Autodesk Inventor part; units mm, degrees
ref_plane "YZ Plane" through (0, 0, 0) normal (1, 0, 0) x (0, 1, 0)
ref_plane "XZ Plane" through (0, 0, 0) normal (0, 1, 0) x (-1, 0, 0)
ref_plane "XY Plane" through (0, 0, 0) normal (0, 0, 1) x (1, 0, 0)
sketch "Sketch1" plane through (0, 0, 0) normal (0, 0, 1) x (1, 0, 0)
  circle A0 centre (0, 0) radius 11.5
  circle A1 centre (-15.5, 15.5) radius 1.5
  circle A2 centre (-15.5, -15.5) radius 1.5
  circle A3 centre (15.5, 15.5) radius 1.5
  circle A4 centre (15.5, -15.5) radius 1.5
  line L0 (-21, -24) -> (21, -24)
  line L1 (0, 20) -> (4.5462, 20) construction
  line L2 (-21, 21) -> (-1, 21)
  line L3 (1, 21) -> (21, 21)
  line L4 (-21, 21) -> (-21, 5.9161)
  line L5 (-21, -5.9161) -> (-21, -24)
  line L6 (21, 21) -> (21, 5.9161)
  line L7 (21, -5.9161) -> (21, -24)
  line L8 (-1.865, 21) -> (1.6498, 21)
  line L9 (-21, 8.451) -> (-21, -8.8551)
  line L10 (21, 10.9387) -> (21, -8.8551)
  dimension "d0" = 23
  dimension "d1" = 3
  dimension "d2" = 3
  dimension "d3" = 24
  dimension "d4" = 8.5
extrude "Extrusion1" add sketch "Sketch1" along normal blind 4
properties part number "StepperHolderTop"
Input: part model. Units: mm. Frame: model coordinates. Give positions to 0.01 mm unless a question says otherwise; leave off trailing zeros. Loops run counter-clockwise (first coordinate to the right, second up) from the corner with the lowest first, then second, coordinate; pieces in that order, holes last. Notation, with made-up numbers: (-23.5, 30.5) - (35.5, 30.5) arc R25 ccw to (35.5, 62.5) - close; hole circle Ø10 at (89, -40). An arc over 180 degrees is marked (long way). Use CSV: the item, a comma, the result in double quotes. Start each with the question number.
Item 1: Section C-C on z = 1.65. Return loops of the section in (x, y), then the cut area to 3 significant figures.
Item 2: Mould query, pull axis Y, two halves, no side actions, for faces 1 (the flat face through (4, -11, 0)), 2 (the flat face through (0, -24, 2)), 3 (the cylindrical face through (-17, -15.57, 1.97)). Classes: pulls with the +Y half, pulls with the -Y half, needs draft (parallel to the pull), parting line crosses it, or undercut.
Item 3: Section B-B on y = -11. Return loops of the section in (x, z), then the cut area to 3 significant figures.
Item 4: Section A-A on x = 0. Return loops of the section in (y, z), then the cut area to 3 significant figures.
Item 5: Section D-D on x = 14.5. Return loops of the section in (y, z), then the cut area to 3 significant figures.
Item 6: Line query: line 1 (Y direction, x = 15.5, z = 1.8); line 2 (X direction, y = -14.5, z = 0.8); line 3 (X direction, y = -8, z = 1.6). Output: solid intervals per line, ascending.
Ans:
1,outline,"(-21, -24) - (21, -24) - (21, 21) - (-21, 21) - close; hole circle Ø3 at (-15.5, -15.5); hole circle Ø3 at (-15.5, 15.5); hole circle Ø23 at (0, 0); hole circle Ø3 at (15.5, -15.5); hole circle Ø3 at (15.5, 15.5)"
1,area,"1,450 mm2"
2,face 1,"needs draft"
2,face 2,"pulls with the -Y half"
2,face 3,"undercut"
3,outline,"(-21, 0) - (-3.35, 0) - (-3.35, 4) - (-21, 4) - close; (3.35, 0) - (21, 0) - (21, 4) - (3.35, 4) - close"
3,area,"141 mm2"
4,outline,"(-24, 0) - (-11.5, 0) - (-11.5, 4) - (-24, 4) - close; (11.5, 0) - (21, 0) - (21, 4) - (11.5, 4) - close"
4,area,"88.0 mm2"
5,outline,"(-24, 0) - (-16.62, 0) - (-16.62, 4) - (-24, 4) - close; (-14.38, 0) - (14.38, 0) - (14.38, 4) - (-14.38, 4) - close; (16.62, 0) - (21, 0) - (21, 4) - (16.62, 4) - close"
5,area,"162 mm2"
6,line 1,"y = -24 to -17, -14 to 14, 17 to 21"
6,line 2,"x = -21 to -16.62, -14.38 to 14.38, 16.62 to 21"
6,line 3,"x = -21 to -8.26, 8.26 to 21"
